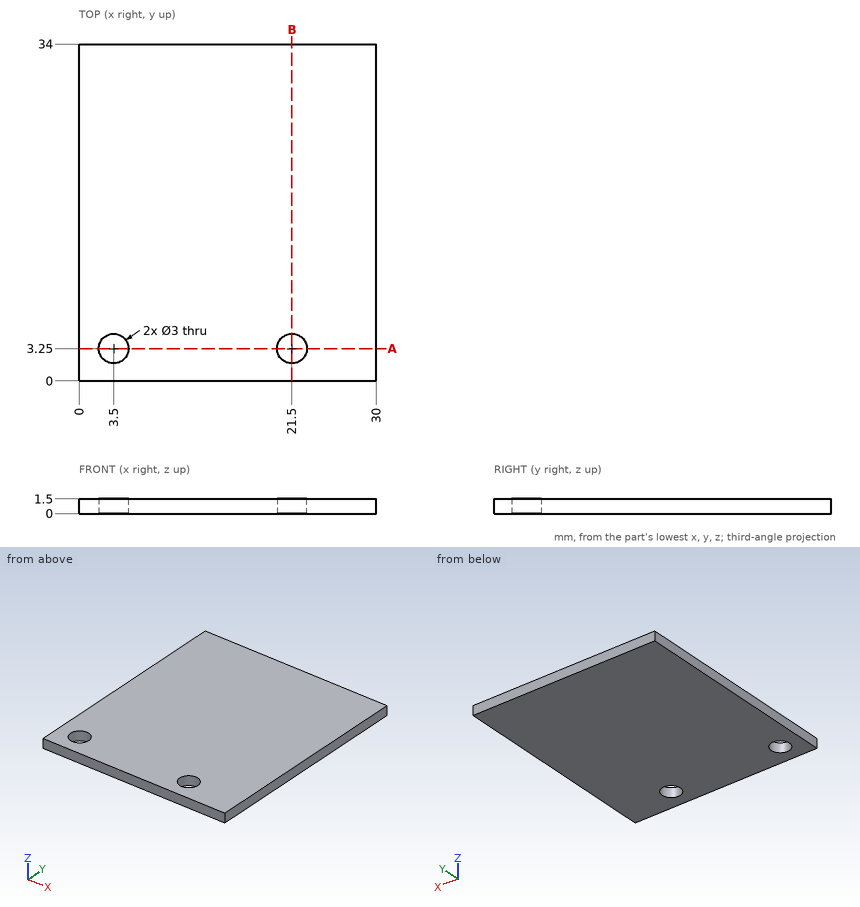
Answer from the drawing. Dimensions are ordinates in mm from the lowest x, y and z of the part. Give positions to 0.01 mm unless a question says otherwise; leave off trailing zeros. Loops run counter-clockwise (first coordinate to the right, second up) from the corner with the lowest first, then second, coordinate; pieces in that order, holes last. Notation, with made-up numbers: (62.25, 57) - (66.25, 57) arc R22 ccw to (66.25, 69) - close; hole circle Ø5 at (21, 89). An arc over 180 degrees is marked (long way). Answer as CSV lines item,"result". Start each with the question number.
Item 1: A cutting plane is placed at B-B on x = 21.5. Determine the outline of the cut face in (y, z).
Item 2: A cutting plane is placed at A-A on y = 3.25. Determine the outline of the cut face in (x, z), then the cut area to 3 significant figures.
Item 3: Find the intervals of material crossed by line 1 (X direction, y = 3.25, z = 0.9); line 2 (Y direction, x = 3.5, z = 0.9); line 3 (Y direction, x = 2.5, z = 0.2), in increasing order. Write a range as from..to.
Found:
1,outline,"(0, 0) - (1.75, 0) - (1.75, 1.5) - (0, 1.5) - close; (4.75, 0) - (34, 0) - (34, 1.5) - (4.75, 1.5) - close"
2,outline,"(0, 0) - (2, 0) - (2, 1.5) - (0, 1.5) - close; (5, 0) - (20, 0) - (20, 1.5) - (5, 1.5) - close; (23, 0) - (30, 0) - (30, 1.5) - (23, 1.5) - close"
2,area,"36.0 mm^2"
3,line 1,"x = 0..2, 5..20, 23..30"
3,line 2,"y = 0..1.75, 4.75..34"
3,line 3,"y = 0..2.13, 4.37..34"
